Design review of the part built by this model. Coordinates are the model's own, in mm. Give positions to 0.01 mm unless a question says otherwise; leave off trailing zeros. Loops run counter-clockwise (first coordinate to the right, second up) from the corner with the lowest first, then second, coordinate; pieces in that order, holes last. Notation, with made-up numbers: M -10,58.25 L 31,58.25 A22 cw 31,97.25 Z; hole C 28.25,-10 d11. An arc over 180 degrees is marked long. Use CSV: the item, a comma, the result in double quotes.
from build123d import *

# Parameters (mm, degrees)
F0_R     = 10.135287
F1_DEPTH = 2
F3_DEPTH = 1
F4_R     = 10.135287
F4_R_2   = 9.5
F5_DEPTH = 1


with BuildPart() as f1:
    # F0 (on Top) → F1 (new body)
    with BuildSketch(Plane.XY):
        Circle(F0_R)
    extrude(amount=-F1_DEPTH)

    # F2 (on face) → F3 (join)
    with BuildSketch(Plane.XY):
        Polygon((6.441801, -5.260301), (3.496772, 1.665972), (2.287066, 0.456266), (4.44094, -5.260301), align=None)
        Polygon((0, 6.526335), (1.786038, 1.786038), (2.950567, 2.950567), (1.171237, 7.135287), (-1.171237, 7.135287), (-2.950567, 2.950567), (-1.786038, 1.786038), align=None)
        Polygon((-2.287066, 0.456266), (-3.496772, 1.665972), (-6.441801, -5.260301), (-4.44094, -5.260301), align=None)
        Polygon((1.786038, 1.786038), (0, 0), (-1.786038, 1.786038), (-2.950567, 2.950567), (-4.034347, 4.034347), (-4.949747, 3.118947), (-3.496772, 1.665972), (-2.287066, 0.456266), (0, -1.8308), (2.287066, 0.456266), (3.496772, 1.665972), (4.949747, 3.118947), (4.034347, 4.034347), (2.950567, 2.950567), align=None)
    extrude(amount=F3_DEPTH)

    # F4 (on face) → F5 (join)
    with BuildSketch(Plane.XY):
        Circle(F4_R)
        Circle(F4_R_2, mode=Mode.SUBTRACT)
    extrude(amount=F5_DEPTH)


solid = f1.part
(1) Wall thickness on line 1 along X through (y, z) = (2.75, 0.85); line 2 along X through (y, z) = (-1.5, 0.1); line 3 along Y through (x, z) = (5.25, 0.7): over which ranges is each line inside the solid? List them lowest first. Write a range as [from, to].
A:
line 1,"[-9.76, -9.09], [-4.58, -1.42], [1.42, 4.58], [9.09, 9.76]"
line 2,"[-10.02, -9.38], [-4.84, -3.02], [-0.33, 0.33], [3.02, 4.84], [9.38, 10.02]"
line 3,"[-8.67, -7.92], [-5.26, -2.46], [7.92, 8.67]"
(2) The part is to be moulded in two halves that separate along Y. For faces 1 (the flat face through (4.21, 2.38, 0.49)), 2 (the flat face through (0, 0, -2)), 3 (the flat face through (-2.05, 5.07, 0.49)), say which applies: released by +Y, released by -Y, zero draft, split by the parting line, or undercut.
A:
face 1,"undercut"
face 2,"zero draft"
face 3,"undercut"
(3) Clearance check with flat-ended pins moving along their axes: P1, Ø0.8, axis at x = -6, z = 0.5, coming from the -Y side; P2, Ø0.5, axis at x = -0.5, z = 0.5, coming from the +Y side; P3, Ø6, axis at x = 6.5, y = 6, coming from the +Z side; P4, Ø1.5, axis at y = 6, z = 0.5, coming from the -X side. State where each tip first meets the part, or that it passes through.
A:
P1,"y = -8.45"
P2,"y = 10.13"
P3,"z = 1"
P4,"x = -8.67"
(4) We need section A-A on z = 0.4. State the section outline as (x, y) points.
A:
outline,"C 0,0 d20.27; M -6.44,-5.26 L -4.44,-5.26 L -2.29,0.46 L 0,-1.83 L 2.29,0.46 L 4.44,-5.26 L 6.44,-5.26 L 3.5,1.67 L 4.95,3.12 L 4.03,4.03 L 2.95,2.95 L 1.17,7.14 L -1.17,7.14 L -2.95,2.95 L -4.03,4.03 L -4.95,3.12 L -3.5,1.67 Z; hole C 0,0 d19; hole M -1.79,1.79 L 0,0 L 1.79,1.79 L 0,6.53 Z"
(5) We need section D-D on z = -1.1. State the section outline as (x, y) points.
A:
outline,"C 0,0 d20.27"
(6) We need section C-C on y = -0.75. State the section outline as (x, z) points, then the cut area to 3 significant figures.
A:
outline,"M -10.11,-2 L 10.11,-2 L 10.11,1 L 9.47,1 L 9.47,0 L 4.52,0 L 4.52,1 L 2.74,1 L 2.74,0 L 1.08,0 L 1.08,1 L -1.08,1 L -1.08,0 L -2.74,0 L -2.74,1 L -4.52,1 L -4.52,0 L -9.47,0 L -9.47,1 L -10.11,1 Z"
area,"47.4 mm²"
(7) We need section B-B on x = -8.25. State the section outline as (y, z) points, then the cut area to 3 significant figures.
A:
outline,"M -5.89,-2 L 5.89,-2 L 5.89,1 L 4.71,1 L 4.71,0 L -4.71,0 L -4.71,1 L -5.89,1 Z"
area,"25.9 mm²"
